For this review, take the finished solid that the model builds, in its own axes (mm). Face numbers are marked on the shaded views. A direction names the side the tool comes from. Give positions to 0.01 mm unless a question says otherwise; leave off trailing zeros. Loops run counter-clockwise (first coordinate to the right, second up) from the corner with the lowest first, then second, coordinate; pieces in that order, holes last.
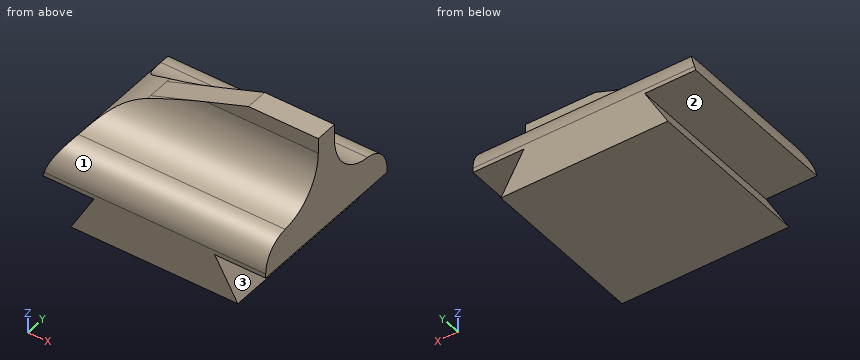
```python
from build123d import *

# Parameters (mm, degrees)
F0_W         = 9.525
F0_H         = 9.525
F1_DEPTH     = 2.286
F2_T1_DEPTH  = 21.3619144247
F3_W         = 2.9083
F3_H         = 9.525
F3_W_2       = 6.8834
F4_DEPTH     = 1.905
F5_R         = 1.6556676611
F6_W         = 12.7
F6_H         = 1.27
F7_DEPTH     = 3.683
F8_SIZE2     = 8.7232408068
F8_SIZE      = 3.175
F9_T4_DEPTH  = 12.7
F9_T9_DEPTH  = 12.7
F10_T1_DEPTH = 20.6733949541


# Not quite as in the source:
# - a fillet or chamfer that OpenCascade refuses, or shapes differently, is made with other operations: its cross-section is extruded or revolved along the edge and cut away or added


with BuildPart() as f1:
    # F0 (on Top) → F1 (new body)
    with BuildSketch(Plane.XY):
        Rectangle(F0_W, F0_H)
    extrude(amount=F1_DEPTH)

    # F2: chamfer of 1.3208 x 2.2876927066 on 2 edges, made by hand

    # F2_s2 → F2_t1 (cut)
    with BuildSketch(Plane.XZ.offset(-10.6809572123)):
        Polygon((-4.7625, -0.0016927066), (-3.4417, 2.286), (-4.7625, 2.286), align=None)
        Polygon((4.7625, -0.0016927066), (3.4417, 2.286), (4.7625, 2.286), align=None)
    extrude(amount=F2_T1_DEPTH, mode=Mode.SUBTRACT)

    # F3 (on face) → F4 (join)
    with BuildSketch(Plane.XY.offset(2.286)):
        with Locations((4.89585, 0)):
            Rectangle(F3_W, F3_H)
        Rectangle(F3_W_2, F3_H)
        with Locations((-4.89585, 0)):
            Rectangle(F3_W, F3_H)
    extrude(amount=F4_DEPTH)

    # F5
    f5_edges = [f1.edges().sort_by_distance(p)[0] for p in [
        (0, 4.7625, 4.191),
        (0, -4.7625, 4.191),
    ]]
    fillet(f5_edges, radius=F5_R)

    # F6 (on face) → F7 (join)
    with BuildSketch(Plane.XY.offset(4.191)):
        Rectangle(F6_W, F6_H)
    extrude(amount=F7_DEPTH)

    # F8
    f8_edges = [f1.edges().sort_by_distance(p)[0] for p in [
        (-6.35, 0, 7.874),
    ]]
    f8_side = f1.faces().sort_by_distance((-6.35, 0, 3.810575))[0]
    chamfer(f8_edges, length=F8_SIZE, length2=F8_SIZE2, reference=f8_side)

    # F9: fillet of radius 2.8207671263 on 2 edges, made by hand


with BuildPart() as f9_tool2:
    # F9_s3 → F9_t4 (new body)
    with BuildSketch(Plane.YZ.offset(-6.35)):
        with BuildLine():
            ThreePointArc((-0.635, 6.9981468006), (-1.3849039981, 5.0828783899), (-3.235890411, 4.1859623453))
            Line((-3.235890411, 4.1859623453), (-3.2139027394, 3.9047438998))
            ThreePointArc((-3.2139027394, 3.9047438998), (-3.1068323389, 3.9089232874), (-0.635, 3.9089232874))
            Line((-0.635, 3.9089232874), (-0.3529232874, 4.191))
            Line((-0.3529232874, 4.191), (-0.3529232874, 6.9981468006))
            Line((-0.3529232874, 6.9981468006), (-0.635, 6.9981468006))
        make_face()
    extrude(amount=F9_T4_DEPTH)

    split(bisect_by=Plane(origin=(-2.2530383821, 0, 6.1901720799), x_dir=(0, 1, 0), z_dir=(0.3420201433, 0, -0.9396926208)), keep=Keep.TOP)


with BuildPart() as f1_1:
    add(f1.part)

    # F9_t1: union F9_tool2
    add(f9_tool2.part)


with BuildPart() as f9_tool7:
    # F9_s8 → F9_t9 (new body)
    with BuildSketch(Plane.YZ.offset(6.35)):
        with BuildLine():
            ThreePointArc((0.635, 6.9981468006), (1.3849039981, 5.0828783899), (3.235890411, 4.1859623453))
            Line((3.235890411, 4.1859623453), (3.2139027394, 3.9047438998))
            ThreePointArc((3.2139027394, 3.9047438998), (3.1068323389, 3.9089232874), (0.635, 3.9089232874))
            Line((0.635, 3.9089232874), (0.3529232874, 4.191))
            Line((0.3529232874, 4.191), (0.3529232874, 6.9981468006))
            Line((0.3529232874, 6.9981468006), (0.635, 6.9981468006))
        make_face()
    extrude(amount=-F9_T9_DEPTH)

    split(bisect_by=Plane(origin=(-2.2530383821, 0, 6.1901720799), x_dir=(0, 1, 0), z_dir=(0.3420201433, 0, -0.9396926208)), keep=Keep.TOP)


with BuildPart() as f1_2:
    add(f1_1.part)

    # F9_t6: union F9_tool7
    add(f9_tool7.part)

    # F10: fillet of radius 5.08 on 1 edges, made by hand

    # F10_s2 → F10_t1 (cut)
    with BuildSketch(Plane.XZ.offset(-10.336697477)):
        with BuildLine():
            ThreePointArc((-6.3503887376, 2.2860942499), (-5.1990968175, 4.4769990033), (-3.1494899918, 5.8643160486))
            Line((-3.1494899918, 5.8643160486), (-3.3233118727, 6.3418877414))
            ThreePointArc((-3.3233118727, 6.3418877414), (-4.9234984728, 5.7590417786), (-6.5238218809, 5.1765716928))
            Line((-6.5238218809, 5.1765716928), (-6.8582211803, 4.699))
            ThreePointArc((-6.8582211803, 4.699), (-6.8582211803, 3.492547125), (-6.8443004931, 2.4058437629))
            Line((-6.8443004931, 2.4058437629), (-6.3503887376, 2.2860942499))
        make_face()
    extrude(amount=F10_T1_DEPTH, mode=Mode.SUBTRACT)


solid = f1_2.part
```
Q1. Consider section A-A on x = -4.5. Give the boundary of the cut face in (y, z), plus the area to 3 significant figures.
Answers:
outline: (-4.76, 0) - (4.76, 0) - (4.76, 0.45) - (-4.76, 0.45) - close; (-4.76, 2.29) - (4.76, 2.29) - (4.76, 2.54) arc R1.66 ccw to (3.24, 4.19) arc R2.82 cw to (1.35, 5.12) - (-1.35, 5.12) arc R2.82 cw to (-3.24, 4.19) arc R1.66 ccw to (-4.76, 2.54) - close
area: 25.0 mm2
Q2. Machinability: for the marked faces 1, 2 and 3, which of the approach directions +Z, -Z, +X, -X, +Y, -Y give a long, thin tool a straight path to every point of the face, cutting with its end or side? Answer none if there is none.
Answers:
face 1: +Z, +X, -X, -Y
face 2: -X, +Y, -Y
face 3: +X, +Y, -Y
Q3. For probe 1 along Y at (x, z) = (4.75, 6.5); probe 2 along Y at (x, z) = (-4.75, 4.75); probe 3 along X at (y, z) = (1.5, 4.25), list the stretches that pass through material, from the lowest coordinate up.
Answers:
probe 1: y = -0.68 to 0.68
probe 2: y = -1.75 to 1.75
probe 3: x = -5.39 to 6.35
Q4. Consider section D-D on z = 1.5. Give the boundary of the cut face in (x, y), plus the area to 3 significant figures.
Answers:
outline: (-3.9, -4.76) - (3.9, -4.76) - (3.9, 4.76) - (-3.9, 4.76) - close
area: 74.2 mm2
Q5. Consider section C-C on x = -2.5. Give the boundary of the cut face in (y, z) (1 decimal), plus the area to 3 significant figures.
Answers:
outline: (-4.8, 0) - (4.8, 0) - (4.8, 2.5) arc R1.7 ccw to (3.2, 4.2) arc R2.8 cw to (0.8, 6.1) - (-0.8, 6.1) arc R2.8 cw to (-3.2, 4.2) arc R1.7 ccw to (-4.8, 2.5) - close
area: 44.4 mm2
Q6. For pin 1 Ø3 at (y, z) = (2, 5.5) entering from -X; pin 2 Ø1 at (x, z) = (2.5, 6) entering from +Y; pin 3 Ø1.5 at (y, z) = (-0.5, 1.5) entering from -X; pin 4 Ø2.5 at (x, y) = (5, -0.5) entering from -Z, all flat-tipped, find the tip position at first contact; note any pin that passes through.
Answers:
pin 1: stops at x = -5.58
pin 2: stops at y = 1.07
pin 3: stops at x = -4.33
pin 4: stops at z = 0
